Here's how the part is built. I have some questions about the finished solid (model axes, mm). A direction names the side the tool comes from. Coordinates: 2 decimals unless noted, no trailing zeros. Write each loop counter-clockwise with the first axis right and the second up, starting at its lowest first coordinate (ties: lowest second). Pieces come first, ordered by that corner, then holes. Notation, with made-up numbers: (-33, -31.5) -> (-17, -31.5) arc R9 cw to (-17, -24.5) -> close; hole circle Ø8 at (-17.5, 44). An arc over 180 degrees is marked (long way). Put each result on its own line as item: value.
```python
from build123d import *

# Parameters (mm, degrees)
SKETCH1_R               = 3.81
BOSS_EXTRUDE1_DEPTH     = 22.225
SKETCH2_R               = 6.2865
SKETCH2_R_2             = 3.7465
CUT_EXTRUDE_THIN3_DEPTH = 7.874


with BuildPart() as part:
    # Sketch1 → Boss-Extrude1 (new body, symmetric)
    with BuildSketch(Plane(origin=(0, 0, 0), x_dir=(0, 0, -1), z_dir=(1, 0, 0))):
        Circle(SKETCH1_R)
    extrude(amount=BOSS_EXTRUDE1_DEPTH, both=True)

    # Sketch2 → Cut-Extrude-Thin3 (cut)
    with BuildSketch(Plane(origin=(22.225, 0, 0), x_dir=(0, 0, -1), z_dir=(1, 0, 0))):
        Circle(SKETCH2_R)
        Circle(SKETCH2_R_2, mode=Mode.SUBTRACT)
    cut_extrude_thin3 = extrude(amount=-CUT_EXTRUDE_THIN3_DEPTH, mode=Mode.SUBTRACT)

    # Mirror1: Cut-Extrude-Thin3 across plane
    add(cut_extrude_thin3.mirror(Plane(origin=(0, 0, 0), x_dir=(0, 0, 1), z_dir=(1, 0, 0))), mode=Mode.SUBTRACT)


solid = part.part
```
Item 1: Imagine slicing it at A-A on z = 2.5. Write out the boundary of the cut face in (x, y) (3 decimals).
Output:
outline: (-22.225, -2.79) -> (-14.351, -2.79) -> (-14.351, -2.875) -> (14.351, -2.875) -> (14.351, -2.79) -> (22.225, -2.79) -> (22.225, 2.79) -> (14.351, 2.79) -> (14.351, 2.875) -> (-14.351, 2.875) -> (-14.351, 2.79) -> (-22.225, 2.79) -> close
Item 2: For P1, Ø1.5, axis at x = 7, y = 1, coming from the +Z side; P2, Ø1, axis at x = -4.5, y = 0.5, coming from the -Z side, each with a flat end and sliding along its axis, tell me the tip position at first contact or that it passes through.
Output:
P1: stops at z = 3.8
P2: stops at z = -3.81
Item 3: Which directions (+Z, -Z, +X, -X, +Y, -Y) give clear straight access to the entire face, cutting with the end or side of a thin tool? Please do faces 1 (the cylindrical face through (18.343, 3.715, 0.488)), 2 (the flat face through (-22.225, 0, 0)), 3 (the cylindrical face through (-18.343, 3.715, 0.488)).
Output:
face 1: +X
face 2: +Z, -Z, -X, +Y, -Y
face 3: -X
Item 4: Please list where these lines run through material, in increasing order: line 1 along Y through (x, z) = (-4, -0.25); line 2 along Y through (x, z) = (20, -0.75); line 3 along Z through (x, y) = (14, 2.25). Write a range as from..to.
Output:
line 1: y = -3.8..3.8
line 2: y = -3.67..3.67
line 3: z = -3.07..3.07
Item 5: Imagine slicing it at C-C on x = -2. Write out the boundary of the cut face in (y, z).
Output:
outline: circle Ø7.62 at (0, 0)
Item 6: Imagine slicing it at D-D on x = 18.5. Write out the boundary of the cut face in (y, z).
Output:
outline: circle Ø7.49 at (0, 0)
Item 7: Imagine slicing it at B-B on y = 2.25. Write out the boundary of the cut face in (x, z) (3 decimals), then the cut area to 3 significant figures.
Output:
outline: (-22.225, -2.996) -> (-14.351, -2.996) -> (-14.351, -3.075) -> (14.351, -3.075) -> (14.351, -2.996) -> (22.225, -2.996) -> (22.225, 2.996) -> (14.351, 2.996) -> (14.351, 3.075) -> (-14.351, 3.075) -> (-14.351, 2.996) -> (-22.225, 2.996) -> close
area: 271 mm²
